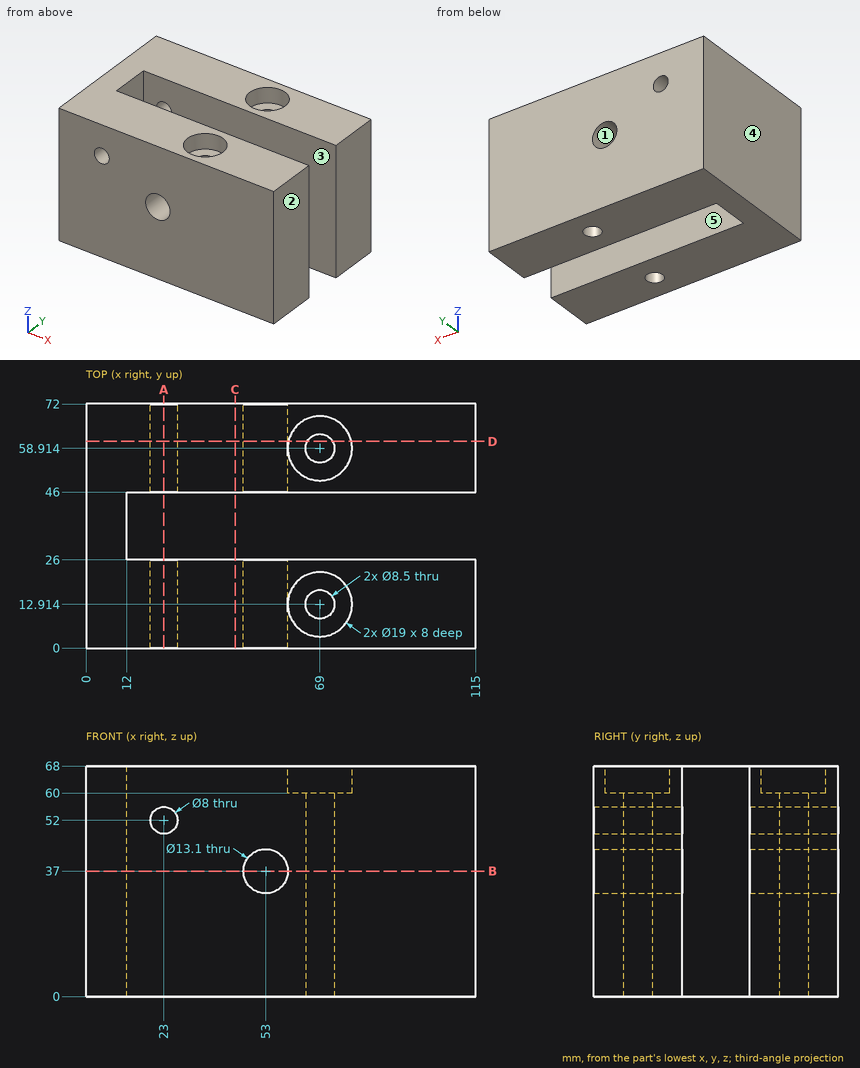
Check sheet for the drawn part. Datum: minimum x, y, z corner. Units: mm. A direction names the side the tool comes from. Round coordinates to 2 decimals unless told otherwise and drop trailing zeros. Loops run counter-clockwise (first coordinate to the right, second up) from the corner with the lowest first, then second, coordinate; pieces in that order, holes last. Notation, with made-up numbers: (60.25, -3) - (95.25, -3) arc R19 ccw to (95.25, 7) - close; hole circle Ø5 at (40.5, -5.5). An arc over 180 degrees is marked (long way). Use one line per item in the form item = value.
1. Section check D-D on y = 61. Record the cut outline in (x, z), and give its area (3 significant figures).
A:
outline = (0, 0) - (65.3, 0) - (65.3, 60) - (59.73, 60) - (59.73, 68) - (0, 68) - close; (72.7, 0) - (115, 0) - (115, 68) - (78.27, 68) - (78.27, 60) - (72.7, 60) - close; hole circle Ø8 at (23, 52); hole circle Ø13.1 at (53, 37)
area = 7,040 mm²
2. Gauge pin test, flat ends, axial feed: pin 1 Ø1.5 at (y, z) = (38, 54.5) entering from +X; pin 2 Ø9.5 at (x, y) = (67, 62) entering from +Z. Record the tip position at first contact, or that the pin passes through.
A:
pin_1 = 12
pin_2 = 60
3. Section check B-B on z = 37. Give the number of separate pieces and of enclosed holes in the cut face.
A:
separate_pieces = 3
enclosed_holes = 2
4. Access from +Z, -Z, +X, -X, +Y, -Y to the whole of each face (thin tool, end or side, straight path). Record for the marked faces 4 and 5.
A:
face_4 = +Z, -Z, -X, +Y, -Y
face_5 = +Z, -Z, +X
5. Scan lines: probe 1 along Y at (x, z) = (69, 62.5) (1 decimal); probe 2 along Y at (x, z) = (69, 26) (1 decimal); probe 3 along Z at (x, y) = (23, 20). Record each from-to range of solid material in increasing order.
A:
probe_1 = 0 to 3.4, 22.4 to 26, 46 to 49.4, 68.4 to 72
probe_2 = 0 to 8.7, 17.2 to 26, 46 to 54.7, 63.2 to 72
probe_3 = 0 to 48, 56 to 68
6. Draft check along X on the marked faces 1, 2 and 3. Enter one of: pulls with the +X half, pulls with the -X half, needs draft (parallel to the pull), parting line crosses it, or undercut.
A:
face_1 = undercut
face_2 = pulls with the +X half
face_3 = needs draft
7. Section check A-A on x = 23. Record the cut outline in (y, z), and give its area (3 significant figures).
A:
outline = (0, 0) - (26, 0) - (26, 48) - (0, 48) - close; (0, 56) - (26, 56) - (26, 68) - (0, 68) - close; (46, 0) - (72, 0) - (72, 48) - (46, 48) - close; (46, 56) - (72, 56) - (72, 68) - (46, 68) - close
area = 3,120 mm²
8. Section check C-C on x = 44. Record the cut outline in (y, z), and give its area (3 significant figures).
A:
outline = (0, 0) - (26, 0) - (26, 68) - (0, 68) - close; (46, 0) - (72, 0) - (72, 68) - (46, 68) - close
area = 3,540 mm²
